Source: CAD feature listing. Evaluate the final solid. Frame: model axes, mm. A direction names the side the tool comes from. Give positions to 0.01 mm unless a question says otherwise; leave off trailing zeros. Loops run counter-clockwise (first coordinate to the right, second up) from the corner with the lowest first, then second, coordinate; pieces in that order, holes last. Notation, with made-up numbers: M 67,45 L 103,45 A27 ccw 103,81 Z; hole C -23,80 d10. An arc over 180 degrees is marked long. Write item = value, one per line.
from build123d import *

# Parameters (mm, degrees)
BOSS_EXTRUDE1_DEPTH = 40
SKETCH2_R           = 4.21
CUT_EXTRUDE1_DEPTH  = 40


with BuildPart() as part:
    # Sketch1 → Boss-Extrude1 (new body)
    with BuildSketch(Plane.XY):
        with BuildLine():
            Line((4, 17.996832295), (-4, 17.996832295))
            Line((-4, 17.996832295), (-4, 14.456832295))
            ThreePointArc((-4, 14.456832295), (0, -15), (4, 14.456832295))
            Line((4, 14.456832295), (4, 17.996832295))
        make_face()
    extrude(amount=BOSS_EXTRUDE1_DEPTH)

    # Sketch2 → Cut-Extrude1 (cut)
    with BuildSketch(Plane.XY.offset(40)):
        Circle(SKETCH2_R)
    extrude(amount=-CUT_EXTRUDE1_DEPTH, mode=Mode.SUBTRACT)


solid = part.part
1. First-contact query: pin 1 Ø2 at (x, z) = (8, 29) entering from -Y; pin 2 Ø10 at (y, z) = (11, 7) entering from +X; pin 3 Ø1.5 at (y, z) = (13, 25) entering from +X. Flat tips, straight axial feed; report the tip coordinate or a pass-through.
Derived:
pin_1 = -13.27
pin_2 = 13.75
pin_3 = 8.66
2. Pull-direction query (X, two-part tool) for faces 1 (the cylindrical face through (4.016, 1.265, 20.28)), 2 (the flat face through (-4, 16, 20)), 3 (the flat face through (0, 5, 0)); classes: +X half, -X half, draft (parallel to the pull), parting line (faces both ways), or undercut.
Derived:
face_1 = undercut
face_2 = -X half
face_3 = draft
3. Material intervals for probe 1 along Y at (x, z) = (0, 10); probe 2 along X at (y, z) = (16.5, 35); probe 3 along Y at (x, z) = (1.5, 16), sorted ascending. Write a range as from..to.
Derived:
probe_1 = -15..-4.21, 4.21..18
probe_2 = -4..4
probe_3 = -14.92..-3.93, 3.93..18
4. Cut plane D-D, the plane y = 11.5. Return the cut outline in (x, z), then the cut area to 3 significant figures.
Derived:
outline = M -9.63,0 L 9.63,0 L 9.63,40 L -9.63,40 Z
area = 770 mm²
5. Cut plane C-C, the plane z = 25. Return the cut outline in (x, y), then the cut area to 3 significant figures.
Derived:
outline = M -4,14.46 A15 ccw long 4,14.46 L 4,18 L -4,18 Z; hole C 0,0 d8.42
area = 677 mm²
6. Cut plane A-A, the plane y = 0. Return the cut outline in (x, z), then the cut area to 3 significant figures.
Derived:
outline = M -15,0 L -4.21,0 L -4.21,40 L -15,40 Z; M 4.21,0 L 15,0 L 15,40 L 4.21,40 Z
area = 863 mm²
7. Cut plane B-B, the plane x = 0. Return the cut outline in (y, z), then the cut area to 3 significant figures.
Derived:
outline = M -15,0 L -4.21,0 L -4.21,40 L -15,40 Z; M 4.21,0 L 18,0 L 18,40 L 4.21,40 Z
area = 983 mm²
8. Reachability of faces 4 (the flat face through (0, 17.997, 20)), 5 (the flat face through (4, 16, 20)) from +Z, -Z, +X, -X, +Y, -Y: full face, straight path, thin tool, end or side. Return the list, or none.
Derived:
face_4 = +Z, -Z, +X, -X, +Y
face_5 = +Z, -Z, +X, +Y
